The listing builds one solid part. Answer for the finished solid, in the listing's coordinates (mm). Coordinates: 2 decimals unless noted, no trailing zeros. Answer as a JSON object with one key per item and string values. Group by question number.
1. Determine the mould class of faces 1 (the face through (-3, -27, -175)), 2 (the face through (3, -5, 2)), 3 (the face through (250, -27, -2)) for opening direction Z: released by +Z, released by -Z, zero draft, split by the parting line, or undercut.
2. Given pin 1 (1.5 mm diameter, centred on x = 194.5, z = 91.5, fed in from +Y); pin 2 (2 mm diameter, centred on x = -49.5, z = 50.5, fed in from -Y), each flat-ended and moving along its own axis, determine where each tip first touches the part or whether it passes through.
3. Straight lines are drawn through the part: L1, parallel to Z at x = 50, y = -44.5; L2, parallel to Y at x = -126.5, z = 101; L3, parallel to Y at x = 14.5, z = -126. For each, find the intervals that lie inside material, in ascending order.
from build123d import *

# Parameters (mm, degrees)
F0_W     = 500
F0_H     = 350
F1_DEPTH = 50
F2_R     = 2
F3_DEPTH = 10
F4_W     = 400
F4_H     = 250
F5_DEPTH = 5
F6_SIZE  = 4.99999


# Not quite as in the source:
# - a fillet or chamfer is up to 0.001 mm smaller than in the source, because OpenCascade refuses the exact size


with BuildPart() as f1:
    # F0 (on Front) → F1 (new body)
    with BuildSketch(Plane.XZ):
        Rectangle(F0_W, F0_H)
    extrude(amount=F1_DEPTH)

    # F2 (on face) → F3 (cut)
    with BuildSketch(Plane.XZ.offset(50)):
        with Locations((-50, 50)):
            Circle(F2_R)
        with Locations((50, 50)):
            Circle(F2_R)
        with Locations((50, -50)):
            Circle(F2_R)
        with Locations((-50, -50)):
            Circle(F2_R)
    extrude(amount=-F3_DEPTH, mode=Mode.SUBTRACT)

    # F4 (on face) → F5 (cut)
    with BuildSketch(Plane(origin=(0, 0, 0), x_dir=(-1, 0, 0), z_dir=(0, 1, 0))):
        Rectangle(F4_W, F4_H)
    extrude(amount=-F5_DEPTH, mode=Mode.SUBTRACT)

    # F6 (size 5 in the source; OpenCascade refuses exactly that, so slightly less here)
    f6_edges = [f1.edges().sort_by_distance(p)[0] for p in [
        (250, 0, 0),
        (0, 0, -175),
        (0, 0, 175),
        (-250, 0, 0),
        (-200, 0, 0),
        (0, 0, -125),
        (200, 0, 0),
        (0, 0, 125),
    ]]
    chamfer(f6_edges, length=F6_SIZE)


solid = f1.part
From the geometry:
{
 "1": {"face 1": "released by -Z", "face 2": "undercut", "face 3": "zero draft"},
 "2": {"pin 1": "stops at y = -5", "pin 2": "stops at y = -40"},
 "3": {"L1": "z = -175 to -52, -48 to 48, 52 to 175", "L2": "y = -50 to -5", "L3": "y = -50 to -4"}
}
